```python
from build123d import *

# Parameters (mm, degrees)
BOSS_EXTRUDE1_DEPTH                            = 3
CSK_FOR_M3_FLAT_HEAD_MACHINE_SCREW1_AT_2_COUNT = 2
CSK_FOR_M3_FLAT_HEAD_MACHINE_SCREW1_AT_2_PITCH = 24.249778845
CSK_FOR_M3_FLAT_HEAD_MACHINE_SCREW1_AT_3_COUNT = 2
CSK_FOR_M3_FLAT_HEAD_MACHINE_SCREW1_AT_3_PITCH = 38.620366786
CSK_FOR_M3_FLAT_HEAD_MACHINE_SCREW1_AT_4_COUNT = 2
CSK_FOR_M3_FLAT_HEAD_MACHINE_SCREW1_AT_4_PITCH = 56.46506966
CSK_FOR_M3_FLAT_HEAD_MACHINE_SCREW1_AT_5_COUNT = 2
CSK_FOR_M3_FLAT_HEAD_MACHINE_SCREW1_AT_5_PITCH = 73.574936218
CSK_FOR_M3_FLAT_HEAD_MACHINE_SCREW1_AT_6_COUNT = 2
CSK_FOR_M3_FLAT_HEAD_MACHINE_SCREW1_AT_6_PITCH = 69.463901996
CSK_FOR_M3_FLAT_HEAD_MACHINE_SCREW1_AT_7_COUNT = 2
CSK_FOR_M3_FLAT_HEAD_MACHINE_SCREW1_AT_7_PITCH = 110.058179925
CSK_FOR_M3_FLAT_HEAD_MACHINE_SCREW1_AT_8_COUNT = 2
CSK_FOR_M3_FLAT_HEAD_MACHINE_SCREW1_AT_8_PITCH = 79.426938293
CSK_FOR_M3_FLAT_HEAD_MACHINE_SCREW1_AT_9_COUNT = 2
CSK_FOR_M3_FLAT_HEAD_MACHINE_SCREW1_AT_9_PITCH = 113.158637276
CSK_FOR_M3_FLAT_HEAD_MACHINE_SCREW1_AT_1_COUNT = 2
CSK_FOR_M3_FLAT_HEAD_MACHINE_SCREW1_AT_1_PITCH = 121.80851999
CSK_FOR_M3_FLAT_HEAD_MACHINE_SCREW1_2_COUNT    = 2
CSK_FOR_M3_FLAT_HEAD_MACHINE_SCREW1_2_PITCH    = 110.121224394
CSK_FOR_M3_FLAT_HEAD_MACHINE_SCREW1_3_COUNT    = 2
CSK_FOR_M3_FLAT_HEAD_MACHINE_SCREW1_3_PITCH    = 124.350346483
HOLE1_D                                        = 7
HOLE2_D                                        = 8
CUT_EXTRUDE1_DEPTH                             = 4


with BuildPart() as part:
    # Sketch2 → Boss-Extrude1 (new body)
    with BuildSketch(Plane.ZY.offset(20)):
        with BuildLine():
            Line((-20.652022209, 137.058847244), (48.554021991, 101.961148745))
            ThreePointArc((48.554021991, 101.961148745), (54.55162088, 96.432765529), (56.769427994, 88.583208534))
            Line((56.769427994, 88.583208534), (56.769427994, 55.934497609))
            ThreePointArc((56.769427994, 55.934497609), (52.615538646, 44.799981854), (42.183846688, 39.106824497))
            Line((42.183846688, 39.106824497), (27.5, 37))
            Line((27.5, 37), (-27.5, 37))
            Line((-27.5, 37), (-49.95644752, 46.524072909))
            ThreePointArc((-49.95644752, 46.524072909), (-55.128189361, 49.472265428), (-59.475441909, 53.539223516))
            Line((-59.475441909, 53.539223516), (-73.824664919, 70.516397068))
            ThreePointArc((-73.824664919, 70.516397068), (-75.841855651, 74.366160521), (-76.03531425, 78.708085309))
            Line((-76.03531425, 78.708085309), (-69.026291478, 118.458228724))
            ThreePointArc((-69.026291478, 118.458228724), (-67.359474123, 122.47213667), (-64.147238229, 125.399811115))
            Line((-64.147238229, 125.399811115), (-44.856843921, 136.445412513))
            ThreePointArc((-44.856843921, 136.445412513), (-32.831883634, 139.808163597), (-20.652022209, 137.058847244))
        make_face()
    extrude(amount=BOSS_EXTRUDE1_DEPTH)

    # Sketch4 → CSK for M3 Flat Head Machine Screw1 (revolve, cut)
    with BuildSketch(Plane(origin=(-23, 109.419717404, -64.490716019), x_dir=(0, 0, 1), z_dir=(0, 1, 0))):
        Polygon((0, 0), (0, 3), (1.7, 3), (1.7, 1.45), (3.15, 0), align=None)
    csk_for_m3_flat_head_machine_screw1 = revolve(axis=Axis((-29.35, 109.419717404, -64.490716019), (1, 0, 0)), mode=Mode.SUBTRACT)

    # CSK for M3 Flat Head Machine Screw1 at 2: CSK for M3 Flat Head Machine Screw1 ×2
    with Locations(*[Vector(0, -0.9845475, -0.175117733) * (i * CSK_FOR_M3_FLAT_HEAD_MACHINE_SCREW1_AT_2_PITCH) for i in range(1, CSK_FOR_M3_FLAT_HEAD_MACHINE_SCREW1_AT_2_COUNT)]):
        add(csk_for_m3_flat_head_machine_screw1, mode=Mode.SUBTRACT)

    # CSK for M3 Flat Head Machine Screw1 at 3: CSK for M3 Flat Head Machine Screw1 ×2
    with Locations(*[Vector(0, 0.44936004, 0.893350746) * (i * CSK_FOR_M3_FLAT_HEAD_MACHINE_SCREW1_AT_3_PITCH) for i in range(1, CSK_FOR_M3_FLAT_HEAD_MACHINE_SCREW1_AT_3_COUNT)]):
        add(csk_for_m3_flat_head_machine_screw1, mode=Mode.SUBTRACT)

    # CSK for M3 Flat Head Machine Screw1 at 4: CSK for M3 Flat Head Machine Screw1 ×2
    with Locations(*[Vector(0, -0.918754476, 0.394829347) * (i * CSK_FOR_M3_FLAT_HEAD_MACHINE_SCREW1_AT_4_PITCH) for i in range(1, CSK_FOR_M3_FLAT_HEAD_MACHINE_SCREW1_AT_4_COUNT)]):
        add(csk_for_m3_flat_head_machine_screw1, mode=Mode.SUBTRACT)

    # CSK for M3 Flat Head Machine Screw1 at 5: CSK for M3 Flat Head Machine Screw1 ×2
    with Locations(*[Vector(0, -0.488530597, 0.872546764) * (i * CSK_FOR_M3_FLAT_HEAD_MACHINE_SCREW1_AT_5_PITCH) for i in range(1, CSK_FOR_M3_FLAT_HEAD_MACHINE_SCREW1_AT_5_COUNT)]):
        add(csk_for_m3_flat_head_machine_screw1, mode=Mode.SUBTRACT)

    # CSK for M3 Flat Head Machine Screw1 at 6: CSK for M3 Flat Head Machine Screw1 ×2
    with Locations(*[Vector(0, -0.172037386, 0.985090421) * (i * CSK_FOR_M3_FLAT_HEAD_MACHINE_SCREW1_AT_6_PITCH) for i in range(1, CSK_FOR_M3_FLAT_HEAD_MACHINE_SCREW1_AT_6_COUNT)]):
        add(csk_for_m3_flat_head_machine_screw1, mode=Mode.SUBTRACT)

    # CSK for M3 Flat Head Machine Screw1 at 7: CSK for M3 Flat Head Machine Screw1 ×2
    with Locations(*[Vector(0, -0.612582522, 0.790406638) * (i * CSK_FOR_M3_FLAT_HEAD_MACHINE_SCREW1_AT_7_PITCH) for i in range(1, CSK_FOR_M3_FLAT_HEAD_MACHINE_SCREW1_AT_7_COUNT)]):
        add(csk_for_m3_flat_head_machine_screw1, mode=Mode.SUBTRACT)

    # CSK for M3 Flat Head Machine Screw1 at 8: CSK for M3 Flat Head Machine Screw1 ×2
    with Locations(*[Vector(0, -0.848826845, 0.528670964) * (i * CSK_FOR_M3_FLAT_HEAD_MACHINE_SCREW1_AT_8_PITCH) for i in range(1, CSK_FOR_M3_FLAT_HEAD_MACHINE_SCREW1_AT_8_COUNT)]):
        add(csk_for_m3_flat_head_machine_screw1, mode=Mode.SUBTRACT)

    # CSK for M3 Flat Head Machine Screw1 at 9: CSK for M3 Flat Head Machine Screw1 ×2
    with Locations(*[Vector(0, -0.388704043, 0.921362669) * (i * CSK_FOR_M3_FLAT_HEAD_MACHINE_SCREW1_AT_9_PITCH) for i in range(1, CSK_FOR_M3_FLAT_HEAD_MACHINE_SCREW1_AT_9_COUNT)]):
        add(csk_for_m3_flat_head_machine_screw1, mode=Mode.SUBTRACT)

    # CSK for M3 Flat Head Machine Screw1 at 1: CSK for M3 Flat Head Machine Screw1 ×2
    with Locations(*[Vector(0, -0.517083861, 0.855934741) * (i * CSK_FOR_M3_FLAT_HEAD_MACHINE_SCREW1_AT_1_PITCH) for i in range(1, CSK_FOR_M3_FLAT_HEAD_MACHINE_SCREW1_AT_1_COUNT)]):
        add(csk_for_m3_flat_head_machine_screw1, mode=Mode.SUBTRACT)

    # CSK for M3 Flat Head Machine Screw1  2: CSK for M3 Flat Head Machine Screw1 ×2
    with Locations(*[Vector(0, -0.485694017, 0.874128893) * (i * CSK_FOR_M3_FLAT_HEAD_MACHINE_SCREW1_2_PITCH) for i in range(1, CSK_FOR_M3_FLAT_HEAD_MACHINE_SCREW1_2_COUNT)]):
        add(csk_for_m3_flat_head_machine_screw1, mode=Mode.SUBTRACT)

    # CSK for M3 Flat Head Machine Screw1  3: CSK for M3 Flat Head Machine Screw1 ×2
    with Locations(*[Vector(0, -0.430117175, 0.90277307) * (i * CSK_FOR_M3_FLAT_HEAD_MACHINE_SCREW1_3_PITCH) for i in range(1, CSK_FOR_M3_FLAT_HEAD_MACHINE_SCREW1_3_COUNT)]):
        add(csk_for_m3_flat_head_machine_screw1, mode=Mode.SUBTRACT)

    # Hole1 (through all)
    with Locations(Plane.ZY.offset(23)):
        with Locations((-40, 70)):
            Hole(HOLE1_D / 2)

    # Hole2 (through all)
    with Locations(Plane.ZY.offset(23)):
        with Locations((39.769427994, 55.934497609)):
            Hole(HOLE2_D / 2)

    # Sketch10 → Cut-Extrude1 (cut, through all)
    with BuildSketch(Plane.ZY.offset(23)):
        with BuildLine():
            Line((-17.492124963, 50.799855174), (-16.102939542, 58.678317198))
            ThreePointArc((-16.102939542, 58.678317198), (-14.365255646, 59.895056561), (-13.148516283, 58.157372665))
            Line((-13.148516283, 58.157372665), (-14.537701704, 50.278910641))
            ThreePointArc((-14.537701704, 50.278910641), (-16.2753856, 49.062171278), (-17.492124963, 50.799855174))
        make_face()
    extrude(amount=-CUT_EXTRUDE1_DEPTH, mode=Mode.SUBTRACT)


solid = part.part
```
Input: part model. Units: mm. Frame: model coordinates. Round coordinates to 2 decimals unless told otherwise and drop trailing zeros. Loops run counter-clockwise (first coordinate to the right, second up) from the corner with the lowest first, then second, coordinate; pieces in that order, holes last. Notation, with made-up numbers: (82.25, 74.25) -> (127.25, 74.25) arc R22 ccw to (127.25, 99.25) -> close; hole circle Ø5 at (29, -12). An arc over 180 degrees is marked (long way). Write each question's results on one line, items separated by ' | '.
1. Ray query, line 1 (Z direction, x = -22.75, y = 72.5); line 2 (Z direction, x = -22.05, y = 71.5); line 3 (Y direction, x = -20.5, z = -16). Return the intervals inside material, ascending. Write a range as from..to.
Geometry results:
line 1: -75.13..-42.45, -37.55..-3.02, 2.44..56.77 | line 2: -74.56..-43.16, -36.84..-1.26, 0.67..56.77 | line 3: 37..49.04, 59.02..134.7
2. Section A-A (z = 22.5). Return loops of the section in (x, y).
Geometry results:
outline: (-23, 37) -> (-20, 37) -> (-20, 40.3) -> (-21.55, 40.3) -> (-23, 38.85) -> close; (-23, 45.15) -> (-21.55, 43.7) -> (-20, 43.7) -> (-20, 115.17) -> (-23, 115.17) -> close
3. Mould query, pull axis Z, two halves, no side actions, for faces 1 (the face through (-20.786, 57.443, 48.554)), 2 (the face through (-21.479, 122.422, -67.395)), 3 (the face through (-21, 72, 56.769)). Classes: +Z half, -Z half, draft (parallel to the pull), parting line (faces both ways), or undercut.
Geometry results:
face 1: undercut | face 2: -Z half | face 3: +Z half
4. Section C-C (z = -22.5). Return loops of the section in (x, y).
Geometry results:
outline: (-23, 37) -> (-20, 37) -> (-20, 40.3) -> (-21.55, 40.3) -> (-23, 38.85) -> close; (-23, 45.15) -> (-21.55, 43.7) -> (-20, 43.7) -> (-20, 137.91) -> (-23, 137.91) -> close
5. First-contact query: P1, Ø5.5, axis at y = 65.43, z = 39.77, coming from the -X side; P2, Ø2, axis at y = 126.77, z = -29.99, coming from the -X side; P3, Ø4, axis at y = 73.48, z = -0.29, coming from the -X side (3 decimals); P4, Ø4.5, axis at y = 97.47, z = 3.94, coming from the -X side. Flat tips, straight axial feed; report the tip coordinate or a pass-through.
Geometry results:
P1: x = -22.6 | P2: through | P3: x = -21.855 | P4: x = -22.1
6. Section B-B (x = -20.7). State how many separate pieces and enclosed holes the cut face has, and give its area (3 significant figures).
Geometry results:
separate pieces: 1 | enclosed holes: 15 | area: 10,300 mm2
